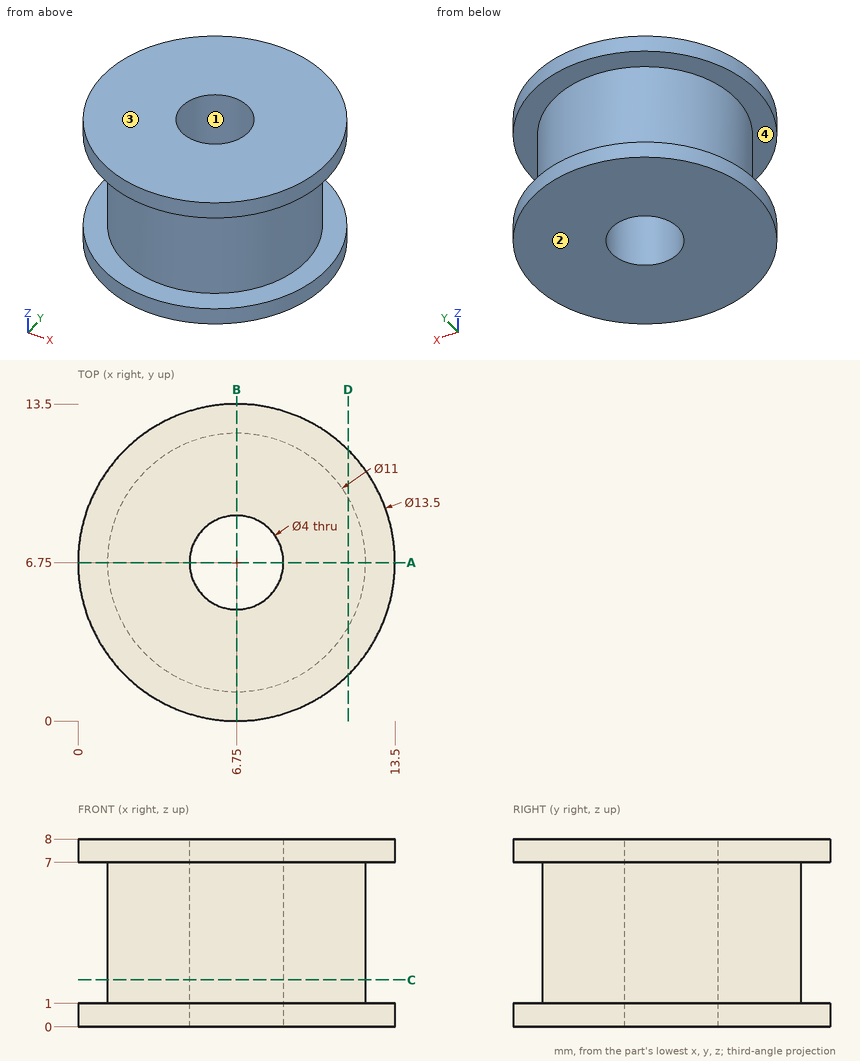
Here's the drawing with two shaded views (mm, measured from the low corner). I have some questions. Coordinates: 2 decimals unless noted, no trailing zeros. Loops run counter-clockwise (first coordinate to the right, second up) from the corner with the lowest first, then second, coordinate; pieces in that order, holes last. Notation, with made-up numbers: M 78.5,-13 L 97.5,-13 A19 cw 97.5,22 Z; hole C 33,17 d2. An arc over 180 degrees is marked long. Put each result on its own line as item: value. Start each with the question number.
(1) We'd pull the mould along Z, two halves only. Please class the marked faces 1, 2, 3 and 4: +Z half, -Z half, draft (parallel to the pull), parting line (faces both ways), or undercut.
(2) Imagine slicing it at D-D on x = 11.5. List the corners of the cut face in (y, z) for me.
(3) Will these pins go through, and if not, where does the flat tip stop? pin 1 Ø1.5 at (x, z) = (7.5, 3.5) entering from +Y; pin 2 Ø2 at (x, z) = (6.5, 3.5) entering from -Y; pin 3 Ø2 at (y, z) = (3, 2.5) entering from +X.
(4) I need wall thicknesses on probe 1 along Y at (x, z) = (6.75, 5.5); probe 2 along Z at (x, y) = (1, 8.5); probe 3 along Y at (x, z) = (7.5, 2). Which ranges of each line are inside material? Lowest first, please.
(5) Imagine slicing it at A-A on y = 6.75. List the corners of the cut face in (x, z) for me.
(6) Imagine slicing it at C-C on z = 2. List the corners of the cut face in (x, y) for me, and give its area (3 significant figures).
Worked answers:
1. face 1: draft
1. face 2: -Z half
1. face 3: +Z half
1. face 4: undercut
2. outline: M 1.95,0 L 11.55,0 L 11.55,1 L 9.52,1 L 9.52,7 L 11.55,7 L 11.55,8 L 1.95,8 L 1.95,7 L 3.98,7 L 3.98,1 L 1.95,1 Z
3. pin 1: stops at y = 12.25
3. pin 2: stops at y = 1.25
3. pin 3: stops at x = 11.51
4. probe 1: y = 1.25 to 4.75, 8.75 to 12.25
4. probe 2: z = 0 to 1, 7 to 8
4. probe 3: y = 1.3 to 4.9, 8.6 to 12.2
5. outline: M 0,0 L 4.75,0 L 4.75,8 L 0,8 L 0,7 L 1.25,7 L 1.25,1 L 0,1 Z; M 8.75,0 L 13.5,0 L 13.5,1 L 12.25,1 L 12.25,7 L 13.5,7 L 13.5,8 L 8.75,8 Z
6. outline: C 6.75,6.75 d11; hole C 6.75,6.75 d4
6. area: 82.5 mm2
